The model under review builds one solid part; all positions refer to its coordinate system, in mm. A direction names the side the tool comes from. Round coordinates to 2 decimals unless told otherwise and drop trailing zeros. Order: outer loops, then holes, each group sorted by start corner. A loop starts at its lowest first (then second) coordinate and runs counter-clockwise, first axis right, second up. Notation, with made-up numbers: M 27,9.5 L 65,9.5 A21 ccw 65,42.5 Z; hole C 33,60 d11. An arc over 180 degrees is marked long. Answer as a JSON object with one key per item and string values. Group by question number.
1. To check wall thickness, follow probe 1 along X at (y, z) = (5.5, 78); probe 2 along Z at (x, y) = (42, 13.5); probe 3 along X at (y, z) = (39, 73). State the ranges of each line that lie inside material, in increasing order. Write a range as [from, to].
2. Machinability: for faces 4 (the face through (-4, 56, 108)), 5 (the face through (1.127, 52.488, 55.82)), which of the approach directions +Z, -Z, +X, -X, +Y, -Y give a long, thin tool a straight path to every point of the face, cutting with its end or side? Answer none if there is none.
3. Add section A-A on x = 0. State the section outline as (y, z) points, and give its area (3 significant figures).
4. Add section B-B on z = 80. State the section outline as (x, y) points, and give its area (3 significant figures).
5. Clearance check with flat-ended pins moving along their axes: P1, Ø8, axis at x = 32, y = 53, coming from the -Z side; P2, Ø3, axis at y = 9, z = 19, coming from the -X side; P3, Ø3, axis at x = -40.5, z = 66.5, coming from the +Y side. State where each tip first meets the part, or that it passes through.
6. Mouldability with a two-part tool opening along X and no side actions: class faces 1 (the face through (-1, 33, 8)), 2 (the face through (1.29, 59.986, 56.835)), 3 (the face through (55, 0, 46)) as released by +X, released by -X, zero draft, split by the parting line, or undercut.
```python
from build123d import *

# Parameters (mm, degrees)
SKETCH_R      = 60
SKETCH_R_2    = 30
PAD_DEPTH     = 8
SKETCH001_R   = 60
SKETCH001_R_2 = 52.5
PAD001_DEPTH  = 100
FILLET_R      = 10
FILLET001_R   = 2
FILLET002_R   = 3
SKETCH002_W   = 200
SKETCH002_H   = 80
POCKET_DEPTH  = 108.001
FILLET003_R   = 2


with BuildPart() as part:
    # Sketch → Pad (new body)
    with BuildSketch(Plane.XY):
        Circle(SKETCH_R)
        Circle(SKETCH_R_2, mode=Mode.SUBTRACT)
    extrude(amount=PAD_DEPTH)

    # Sketch001 (on Face4 of Pad) → Pad001 (join)
    with BuildSketch(Plane.XY.offset(8)):
        Circle(SKETCH001_R)
        Circle(SKETCH001_R_2, mode=Mode.SUBTRACT)
    extrude(amount=PAD001_DEPTH)

    # Fillet
    fillet_edges = [part.edges().sort_by_distance(p)[0] for p in [
        (-60, 0, 0),
    ]]
    fillet(fillet_edges, radius=FILLET_R)

    # Fillet001
    fillet001_edges = [part.edges().sort_by_distance(p)[0] for p in [
        (-30, 0, 0),
        (-30, 0, 8),
    ]]
    fillet(fillet001_edges, radius=FILLET001_R)

    # Fillet002
    fillet002_edges = [part.edges().sort_by_distance(p)[0] for p in [
        (-52.5, 0, 108),
        (-60, 0, 108),
    ]]
    fillet(fillet002_edges, radius=FILLET002_R)

    # Sketch002 (on Face5 of Fillet002) → Pocket (cut, through all)
    with BuildSketch(Plane(origin=(0, 0, 0), x_dir=(1, 0, 0), z_dir=(0, 0, -1))):
        with Locations((0, 40)):
            Rectangle(SKETCH002_W, SKETCH002_H)
    extrude(amount=-POCKET_DEPTH, mode=Mode.SUBTRACT)

    # Fillet003
    fillet003_edges = [part.edges().sort_by_distance(p)[0] for p in [
        (-41, 0, 0),
        (-57.071068, 0, 2.928932),
        (-60, 0, 57.5),
        (-59.12132, 0, 107.12132),
        (-56.25, 0, 108),
        (-53.37868, 0, 107.12132),
        (-52.5, 0, 56.5),
        (-42.25, 0, 8),
        (-30.585786, 0, 7.414214),
        (-30, 0, 4),
        (-30.585786, 0, 0.585786),
        (41, 0, 0),
        (30.585786, 0, 0.585786),
        (30, 0, 4),
        (30.585786, 0, 7.414214),
        (42.25, 0, 8),
        (52.5, 0, 56.5),
        (53.37868, 0, 107.12132),
        (56.25, 0, 108),
        (59.12132, 0, 107.12132),
        (60, 0, 57.5),
        (57.071067, 0, 2.928931),
    ]]
    fillet(fillet003_edges, radius=FILLET003_R)


solid = part.part
```
Recorded:
{
 "1": {"probe 1": "x = [-59.75, -52.21], [52.21, 59.75]", "probe 2": "z = [0, 8]", "probe 3": "x = [-45.6, -35.15], [35.15, 45.6]"},
 "2": {"face 4": "+Z, +X, -X, +Y, -Y", "face 5": "+Z, -Y"},
 "3": {"outline": "M 30,2 A2 ccw 32,0 L 50,0 A10 ccw 60,10 L 60,105 A3 ccw 57,108 L 55.5,108 A3 ccw 52.5,105 L 52.5,8 L 32,8 A2 ccw 30,6 Z", "area": "963 mm²"},
 "4": {"outline": "M -59.96,2.07 A2 ccw -57.97,0 L -54.46,0 A2 ccw -52.46,1.93 A52.5 cw 52.46,1.93 A2 ccw 54.46,0 L 57.97,0 A2 ccw 59.96,2.07 A60 ccw Z", "area": "1,320 mm²"},
 "5": {"P1": "stops at z = 3.88", "P2": "stops at x = -59.53", "P3": "stops at y = 45.6"},
 "6": {"face 1": "undercut", "face 2": "split by the parting line", "face 3": "zero draft"}
}
